from build123d import *

# Parameters (mm, degrees)
SKETCH2_R           = 7
SKETCH2_R_2         = 2
BOSS_EXTRUDE2_DEPTH = 3
SKETCH3_W           = 118.4
SKETCH3_H           = 12.75
CUT_EXTRUDE1_DEPTH  = 338.231374578
SKETCH5_R           = 2.5
SKETCH5_R_2         = 2.306063735
CUT_EXTRUDE2_DEPTH  = 338.231374578


with BuildPart() as part:
    # Sketch2 → Boss-Extrude2 (new body)
    with BuildSketch(Plane.XY):
        with BuildLine():
            Line((25.03035901, 0), (111.286489227, 49.8))
            ThreePointArc((111.286489227, 49.8), (152.858332199, 69.766604349), (181.6, 33.7))
            Line((181.6, 33.7), (181.6, 0))
            Line((181.6, 0), (300, 0))
            Line((300, 0), (300, 145))
            Line((300, 145), (38, 145))
            Line((38, 145), (38, 154))
            Line((38, 154), (19, 154))
            Line((19, 154), (0, 154))
            Line((0, 154), (0, 0))
            Line((0, 0), (25.03035901, 0))
        make_face()
        with Locations((19, 135)):
            Circle(SKETCH2_R, mode=Mode.SUBTRACT)
        with Locations((14, 149.5)):
            Circle(SKETCH2_R_2, mode=Mode.SUBTRACT)
        with Locations(Location((24, 149.5, 0), (0, 0, 180))):
            Circle(SKETCH2_R_2, mode=Mode.SUBTRACT)
    extrude(amount=BOSS_EXTRUDE2_DEPTH)

    # Sketch3 → Cut-Extrude1 (cut, through all)
    with BuildSketch(Plane.XY.offset(3)):
        with Locations((240.8, 6.375)):
            Rectangle(SKETCH3_W, SKETCH3_H)
    extrude(amount=-CUT_EXTRUDE1_DEPTH, mode=Mode.SUBTRACT)

    # Sketch5 → Cut-Extrude2 (cut, through all)
    with BuildSketch(Plane.XY.offset(3)):
        with Locations((254.98, 25.75)):
            Circle(SKETCH5_R)
        with Locations((234.98, 25.75)):
            Circle(SKETCH5_R_2)
    extrude(amount=-CUT_EXTRUDE2_DEPTH, mode=Mode.SUBTRACT)


solid = part.part
Geometry check sheet. Reference: the model listing, model coordinates, mm. Give positions to 0.01 mm unless a question says otherwise; leave off trailing zeros. Loops run counter-clockwise (first coordinate to the right, second up) from the corner with the lowest first, then second, coordinate; pieces in that order, holes last. Notation, with made-up numbers: (-23, -19.75) -> (-8, -19.75) arc R24 cw to (-8, -7.75) -> close; hole circle Ø6 at (44, 48.25). An arc over 180 degrees is marked (long way). Answer in a Markdown table with one row per item. Add a question column.
1) Material ranges on probe 1 along X at (y, z) = (149.5, 1.25); probe 2 along Y at (x, z) = (254.98, 2.4); probe 3 along Y at (x, z) = (234.98, 1.25), recorded low to high. Write a range as from..to.
2) Draft check along X on faces 1 (the face through (67.55, 24.55, 1.48)), 2 (the face through (148, 78, 0)). Enter one of: pulls with the +X half, pulls with the -X half, needs draft (parallel to the pull), parting line crosses it, or undercut.
3) Gauge pin test, flat ends, axial feed: P1, Ø0.9, axis at y = 151, z = 2, coming from the +X side; P2, Ø0.9, axis at x = 259.5, z = 1, coming from the -Y side; P3, Ø5.5, axis at x = 234.98, y = 25.75, coming from the -Z side; P4, Ø11, axis at x = 19, y = 135, coming from the -Z side. Record the tip position at first contact, or that the pin passes through.
4) Cross-section at D-D on x = 206.5. Record the boundary of the cut face in (y, z), and give its area (3 significant figures).
5) Cross-section at C-C on z = 0.7. Record the boundary of the cut face in (x, y).
6) Cross-section at B-B on x = 19. Record the boundary of the cut face in (y, z), and give its area (3 significant figures).
7) Cross-section at A-A on y = 135. Record the boundary of the cut face in (x, z), and give its area (3 significant figures).
Outcome:
| question | item | result |
|---|---|---|
| 1 | probe 1 | x = 0..12, 16..22, 26..38 |
| 1 | probe 2 | y = 12.75..23.25, 28.25..145 |
| 1 | probe 3 | y = 12.75..23.44, 28.06..145 |
| 2 | face 1 | undercut |
| 2 | face 2 | needs draft |
| 3 | P1 | stops at x = 38 |
| 3 | P2 | stops at y = 12.75 |
| 3 | P3 | stops at z = 0 |
| 3 | P4 | passes through |
| 4 | outline | (12.75, 0) -> (145, 0) -> (145, 3) -> (12.75, 3) -> close |
| 4 | area | 397 mm^2 |
| 5 | outline | (0, 0) -> (25.03, 0) -> (111.29, 49.8) arc R37 cw to (181.6, 33.7) -> (181.6, 12.75) -> (300, 12.75) -> (300, 145) -> (38, 145) -> (38, 154) -> (0, 154) -> close; hole circle Ø14 at (19, 135); hole circle Ø4 at (14, 149.5); hole circle Ø4 at (24, 149.5); hole circle Ø4.61 at (234.98, 25.75); hole circle Ø5 at (254.98, 25.75) |
| 6 | outline | (0, 0) -> (128, 0) -> (128, 3) -> (0, 3) -> close; (142, 0) -> (154, 0) -> (154, 3) -> (142, 3) -> close |
| 6 | area | 420 mm^2 |
| 7 | outline | (0, 0) -> (12, 0) -> (12, 3) -> (0, 3) -> close; (26, 0) -> (300, 0) -> (300, 3) -> (26, 3) -> close |
| 7 | area | 858 mm^2 |
